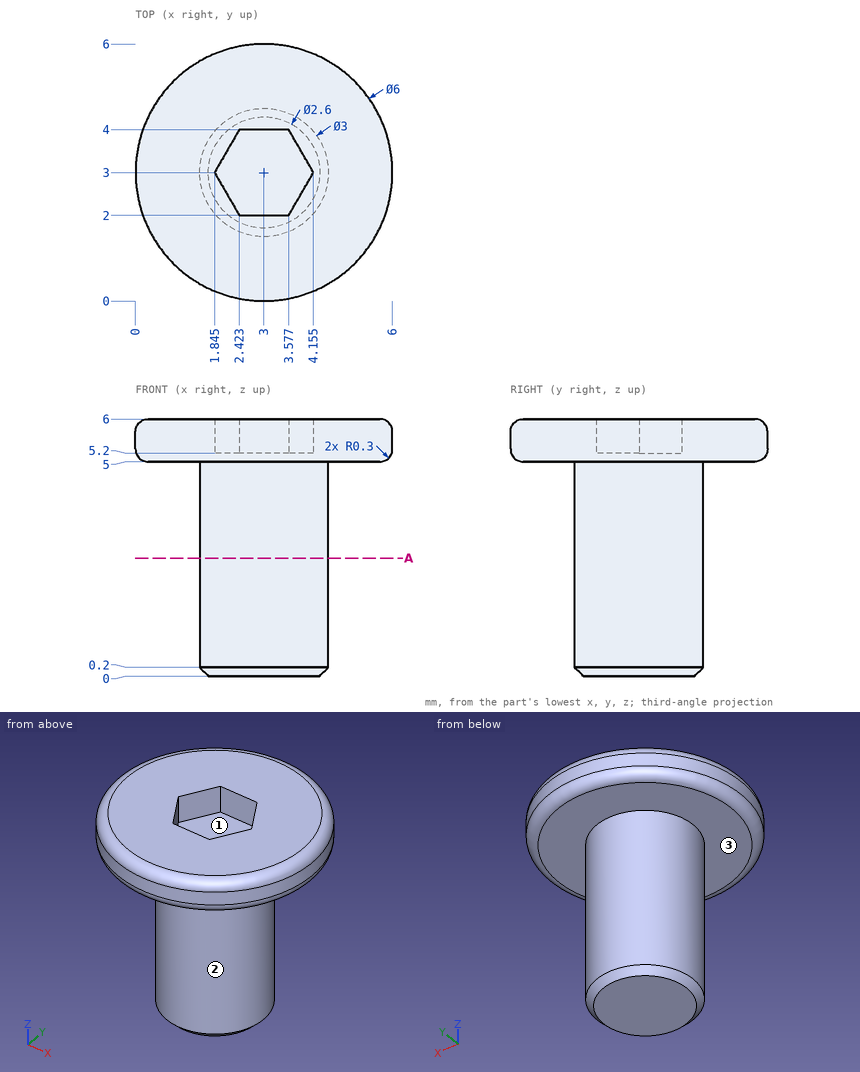
Answer from the drawing. Dimensions are ordinates in mm from the lowest x, y and z of the part. Round coordinates to 2 decimals unless told otherwise and drop trailing zeros. Order: outer loops, then holes, each group sorted by start corner. A loop starts at its lowest first (then second) coordinate and runs counter-clockwise, first axis right, second up.
1) Straight lines are drawn through the part: L1, parallel to X at y = 5.75, z = 5.2 (1 decimal); L2, parallel to X at y = 3.75, z = 4.85; L3, parallel to Z at x = 1, y = 4.75. For each, find the intervals that lie inside material, in ascending order.
2) The mould has two halves that part along Y. Classify the marked faces 1, 2 and 3: released by +Y, released by -Y, zero draft, split by the parting line, or undercut.
3) The part is cut by section A-A on z = 2.75. Write down the section's boundary in (x, y).
4) Flat-ended cylindrical pins translate along their axes: pin 1 (3 mm diameter, centred on y = 3, z = 1.5, fed in from +X); pin 2 (1 mm diameter, centred on x = 3.5, y = 2.5, fed in from +Z). Find the tip coordinate at first contact, or state that the pin passes through.
Resolved:
1. L1: x = 1.8 to 4.2
1. L2: x = 1.7 to 4.3
1. L3: z = 5 to 6
2. face 1: undercut
2. face 2: split by the parting line
2. face 3: zero draft
3. outline: circle Ø3 at (3, 3)
4. pin 1: stops at x = 4.5
4. pin 2: stops at z = 6
